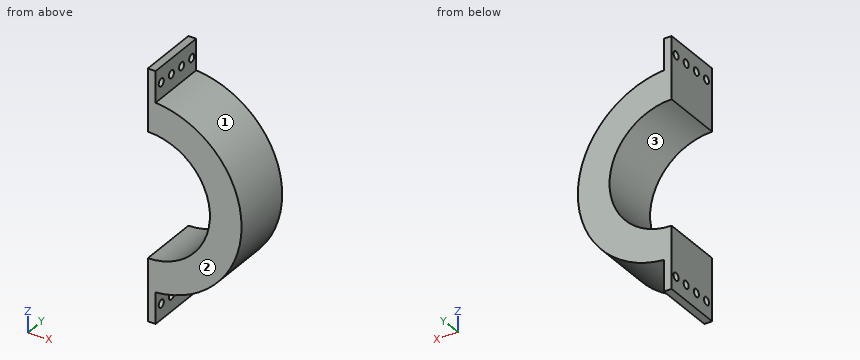
```python
from build123d import *

# Parameters (mm, degrees)
BOSS_EXTRUDE1_DEPTH = 101.6
SKETCH2_R           = 6.35
CUT_EXTRUDE1_DEPTH  = 268.226937902
SKETCH3_R           = 6.35
CUT_EXTRUDE2_DEPTH  = 268.226937902


with BuildPart() as part:
    # Sketch1 → Boss-Extrude1 (new body)
    with BuildSketch(Plane(origin=(0, 0, 0), x_dir=(1, 0, 0), z_dir=(0, 1, 0))):
        with BuildLine():
            Line((0, -101.6), (0, -203.2))
            Line((0, -203.2), (12.7, -203.2))
            Line((12.7, -203.2), (12.7, -152.4))
            ThreePointArc((12.7, -152.4), (153.403362933, 0), (12.7, 152.4))
            Line((12.7, 152.4), (12.7, 203.2))
            Line((12.7, 203.2), (0, 203.2))
            Line((0, 203.2), (0, 101.6))
            ThreePointArc((0, 101.6), (101.6, 0), (0, -101.6))
        make_face()
    extrude(amount=BOSS_EXTRUDE1_DEPTH)

    # Sketch2 → Cut-Extrude1 (cut, through all)
    with BuildSketch(Plane(origin=(12.7, 0, 0), x_dir=(0, 0, -1), z_dir=(1, 0, 0))):
        with Locations((-177.8, 90.380321662)):
            Circle(SKETCH2_R)
        with Locations((-177.8, 64.980321662)):
            Circle(SKETCH2_R)
        with Locations((-177.8, 39.580321662)):
            Circle(SKETCH2_R)
        with Locations((-177.8, 14.180321662)):
            Circle(SKETCH2_R)
    extrude(amount=-CUT_EXTRUDE1_DEPTH, mode=Mode.SUBTRACT)

    # Sketch3 → Cut-Extrude2 (cut, through all)
    with BuildSketch(Plane(origin=(12.7, 0, 0), x_dir=(0, 0, -1), z_dir=(1, 0, 0))):
        with Locations((177.8, 90.380321662)):
            Circle(SKETCH3_R)
        with Locations((177.8, 64.980321662)):
            Circle(SKETCH3_R)
        with Locations((177.8, 39.580321662)):
            Circle(SKETCH3_R)
        with Locations((177.8, 14.180321662)):
            Circle(SKETCH3_R)
    extrude(amount=-CUT_EXTRUDE2_DEPTH, mode=Mode.SUBTRACT)


solid = part.part
```
The listing builds one solid part. Answer for the finished solid, in the listing's coordinates (mm). Face numbers are marked on the shaded views. Give positions to 0.01 mm unless a question says otherwise; leave off trailing zeros. Order: outer loops, then holes, each group sorted by start corner. A loop starts at its lowest first (then second) coordinate and runs counter-clockwise, first axis right, second up. Notation, with made-up numbers: (-21.75, 23.25) -> (13.25, 23.25) arc R20 ccw to (13.25, 50.25) -> close; hole circle Ø8 at (54.25, 23.5). An arc over 180 degrees is marked (long way). Answer as a JSON object with one key per item and string values. Group by question number.
Item 1: Flat-ended cylindrical pins translate along their axes: pin 1 (16.5 mm diameter, centred on y = 14.18, z = -177.8, fed in from +X); pin 2 (6 mm diameter, centred on x = 127, y = 41.5, fed in from -Z); pin 3 (11.5 mm diameter, centred on y = 90.38, z = 177.8, fed in from +X); pin 4 (6 mm diameter, centred on x = 130.5, y = 29.5, fed in from -Z). Find the tip coordinate at first contact, or state that the pin passes through.
Item 2: Determine the mould class of the marked faces 1, 2 and 3 for opening direction Z: pulls with the +Z half, pulls with the -Z half, needs draft (parallel to the pull), parting line crosses it, or undercut.
Item 3: Consider L1, parallel to Y at x = 6, z = -177.8; L2, parallel to Y at x = 3, z = 177; L3, parallel to Z at x = 45.5, y = 24. Determine where each line is inside the solid, lowest interval first. Write a range as from..to.
Item 4: The part is cut by section A-A on z = 177.8. Write down the section's boundary in (x, y).
Item 5: The part is cut by section D-D on z = 0. Write down the section's boundary in (x, y), and give its area (3 significant figures).
Item 6: The part is cut by section C-C on y = 26. Write down the section's boundary in (x, z), and give its area (3 significant figures).
Item 7: The part is cut by section B-B on x = 78.5. Write down the section's boundary in (y, z), and give its area (3 significant figures).
Result set:
{
 "1": {"pin 1": "x = 12.7", "pin 2": "z = -90.15", "pin 3": "through", "pin 4": "z = -85.14"},
 "2": {"face 1": "parting line crosses it", "face 2": "needs draft", "face 3": "undercut"},
 "3": {"L1": "0..7.83, 20.53..33.23, 45.93..58.63, 71.33..84.03, 96.73..101.6", "L2": "0..7.88, 20.48..33.28, 45.88..58.68, 71.28..84.08, 96.68..101.6", "L3": "-146.12..-90.84, 90.84..146.12"},
 "4": {"outline": "(0, 0) -> (12.7, 0) -> (12.7, 7.83) -> (0, 7.83) -> close; (0, 20.53) -> (12.7, 20.53) -> (12.7, 33.23) -> (0, 33.23) -> close; (0, 45.93) -> (12.7, 45.93) -> (12.7, 58.63) -> (0, 58.63) -> close; (0, 71.33) -> (12.7, 71.33) -> (12.7, 84.03) -> (0, 84.03) -> close; (0, 96.73) -> (12.7, 96.73) -> (12.7, 101.6) -> (0, 101.6) -> close"},
 "5": {"outline": "(101.6, 0) -> (153.4, 0) -> (153.4, 101.6) -> (101.6, 101.6) -> close", "area": "5,260 mm²"},
 "6": {"outline": "(0, -203.2) -> (12.7, -203.2) -> (12.7, -152.4) arc R152.89 ccw to (12.7, 152.4) -> (12.7, 203.2) -> (0, 203.2) -> (0, 101.6) arc R101.6 cw to (0, -101.6) -> close", "area": "21,900 mm²"},
 "7": {"outline": "(0, -131.5) -> (101.6, -131.5) -> (101.6, -64.5) -> (0, -64.5) -> close; (0, 64.5) -> (101.6, 64.5) -> (101.6, 131.5) -> (0, 131.5) -> close", "area": "13,600 mm²"}
}
